Autodesk Inventor part; units mm, degrees
ref_plane "Start plane" through (0, 0, 0) normal (0, 0, 1) x (1, 0, 0)
ref_plane "End plane" through (0, 0, 558.8) normal (0, 0, 1) x (1, 0, 0)
ref_plane "Work Plane4" through (1101.598, 19.05, 0) normal (0.7071, 0, 0.7071) x (0.7071, 0, -0.7071)
ref_plane "Start plane" through (0, 0, 0) normal (0, 0, 1) x (1, 0, 0)
ref_plane "End plane" through (0, 0, 558.8) normal (0, 0, 1) x (1, 0, 0)
sketch "Sketch" plane through (0, 0, 0) normal (0, 0, 1) x (1, 0, 0)
  line L0 (38.1, 0) -> (0, 0)
  line L1 (0, 0) -> (0, 38.1)
  line L2 (0, 38.1) -> (2.4765, 38.1)
  line L3 (4.7625, 35.814) -> (4.7625, 9.5885)
  line L4 (9.5885, 4.7625) -> (35.814, 4.7625)
  line L5 (38.1, 2.4765) -> (38.1, 0)
  line L6 (0, -11.0414) -> (0, 31.5385) construction
  line L7 (-11.0414, 0) -> (31.5385, 0) construction
  arc A0 (4.7625, 9.5885) -> (9.5885, 4.7625) centre (9.5885, 9.5885) ccw
  arc A1 (4.7625, 35.814) -> (2.4765, 38.1) centre (2.4765, 35.814) ccw
  arc A2 (38.1, 2.4765) -> (35.814, 4.7625) centre (35.814, 2.4765) ccw
  line L8 (0, 48.4964) -> (0, -20.9644) construction
  line L9 (-20.9644, 0) -> (48.4964, 0) construction
  point P0 (4.7625, 38.1)
  point P1 (4.7625, 4.7625)
  point P2 (38.1, 4.7625)
  dimension "d0" = 38.1
  dimension "d1" = 38.1
  dimension "d2" = 4.7625
  dimension "d3" = 4.7625
  dimension "d10" = 0
  dimension "d11" = 0
  dimension "d14" = 4.826
  dimension "d15" = 2.286
extrude "Body" add sketch "Sketch" along normal up to surface (558.8 mm away) from surface at 0
sketch "Sketch3" plane through (0, 0, 0) normal (0, 0, 1) x (1, 0, 0)
  line L0 (0, 0) -> (10, 0)
ref_plane "Work Plane3" through (0, 0, 0) normal (0, -1, 0) x (1, 0, 0)
sketch "Sketch4" plane through (0, 0, 0) normal (0, -1, 0) x (1, 0, 0)
  line L0 (-2, 0) -> (12, 0)
  line L1 (-2, 558.8) -> (12, 558.8)
  dimension "d17" = 558.8
ref_plane "Work Plane4" through (1101.598, 19.05, 0) normal (0.7071, 0, 0.7071) x (0.7071, 0, -0.7071)
ref_plane "Work Plane5" through (-130.302, 19.05, 0) normal (-0.7071, 0, 0.7071) x (0.7071, 0, 0.7071)
ref_plane "Work Plane6" through (485.648, 0, 0) normal (-1, 0, 0) x (0, 0, 1)
sketch "Sketch5" plane through (485.648, 0, 0) normal (-1, 0, 0) x (0, 0, 1)
  line L0 (38.1, 0) -> (0, 0)
  line L1 (0, 0) -> (0, 38.1)
  line L2 (0, 38.1) -> (2.4765, 38.1)
  arc A0 (4.7625, 35.814) -> (2.4765, 38.1) centre (2.4765, 35.814) ccw
  line L3 (4.7625, 35.814) -> (4.7625, 9.5885)
  arc A1 (4.7625, 9.5885) -> (9.5885, 4.7625) centre (9.5885, 9.5885) ccw
  line L4 (9.5885, 4.7625) -> (35.814, 4.7625)
  arc A2 (38.1, 2.4765) -> (35.814, 4.7625) centre (35.814, 2.4765) ccw
  line L5 (38.1, 2.4765) -> (38.1, 0)
extrude "Extrusion2" cut sketch "Sketch5" along normal up to surface from surface at -615.95 surface through (-130.302, 19.05, 0) normal (-0.7071, 0, 0.7071)
ref_plane "Work Plane7" through (1101.598, 19.05, 558.8) normal (0.7071, 0, -0.7071) x (0, 1, 0)
ref_plane "Work Plane8" through (-130.302, 19.05, 558.8) normal (-0.7071, 0, -0.7071) x (0, 1, 0)
ref_plane "Work Plane9" through (485.648, 0, 558.8) normal (-1, 0, 0) x (0, 1, 0)
sketch "Sketch6" plane through (485.648, 0, 558.8) normal (-1, 0, 0) x (0, 1, 0)
  line L0 (38.1, 0) -> (0, 0)
  line L1 (0, 0) -> (0, 38.1)
  line L2 (0, 38.1) -> (2.4765, 38.1)
  arc A0 (4.7625, 35.814) -> (2.4765, 38.1) centre (2.4765, 35.814) ccw
  line L3 (4.7625, 35.814) -> (4.7625, 9.5885)
  arc A1 (4.7625, 9.5885) -> (9.5885, 4.7625) centre (9.5885, 9.5885) ccw
  line L4 (9.5885, 4.7625) -> (35.814, 4.7625)
  arc A2 (38.1, 2.4765) -> (35.814, 4.7625) centre (35.814, 2.4765) ccw
  line L5 (38.1, 2.4765) -> (38.1, 0)
extrude "Extrusion3" cut sketch "Sketch6" along normal up to surface from surface at -615.95 surface through (-130.302, 19.05, 558.8) normal (-0.7071, 0, -0.7071)
equation "\"d0\" = G_H"
equation "\"d1\" = G_H"
equation "\"d2\" = G_T"
equation "\"d3\" = G_T"
equation "\"d14\" = G_IR"
equation "\"d15\" = G_ER"
equation "\"d4\" = G_L"
equation "\"G_H\" = 38.1"
equation "\"G_T\" = 4.7625"
equation "\"G_ER\" = 2.286"
equation "\"G_IR\" = 4.826"
equation "\"G_L\" = d17"
equation "\"ex\" = 0"
equation "\"G_OFFSET_START\" = 0"
equation "\"G_OFFSET_END\" = 0"
equation "\"d13\" = G_OFFSET_END + B_L"
equation "\"B_L\" = 558.8"
properties part number "AISC - L 1.5 x 1.5 x 3/16 - 22" material "Aluminum 6061"
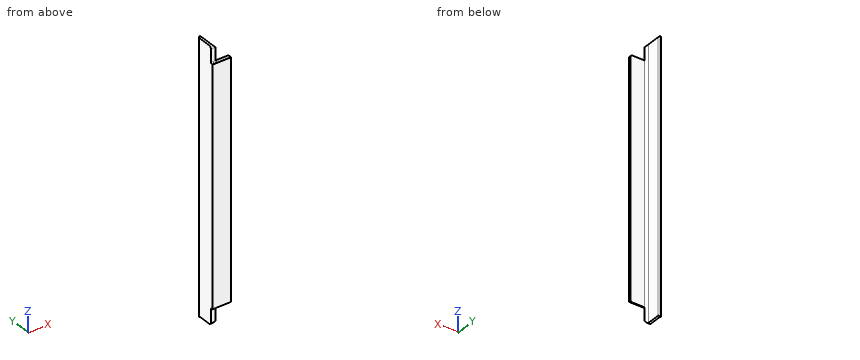
Source: CAD feature listing. Evaluate the final solid. Frame: model axes, mm. Round coordinates to 2 decimals unless told otherwise and drop trailing zeros. Order: outer loops, then holes, each group sorted by start corner. A loop starts at its lowest first (then second) coordinate and runs counter-clockwise, first axis right, second up. Notation, with made-up numbers: (54.25, 25.5) -> (91.25, 25.5) arc R35 cw to (91.25, 59.5) -> close; hole circle Ø2 at (-2.75, -2.5). An arc over 180 degrees is marked (long way). Use CSV: the item, a comma, the result in double quotes.
(1) Section B-B on x = 29. Return the cut outline in (y, z), and give its area (3 significant figures).
Report:
outline,"(0, 38.1) -> (2.48, 38.1) arc R2.29 cw to (4.76, 35.81) -> (4.76, 522.99) arc R2.29 cw to (2.48, 520.7) -> (0, 520.7) -> close"
area,"2,300 mm^2"
(2) Section C-C on y = 28. Return the cut outline in (x, z).
Report:
outline,"(0, 4.76) -> (4.76, 4.76) -> (4.76, 554.04) -> (0, 554.04) -> close"
(3) Section A-A on z = 362.5. Return the cut outline in (x, y).
Report:
outline,"(0, 0) -> (38.1, 0) -> (38.1, 2.48) arc R2.29 ccw to (35.81, 4.76) -> (9.59, 4.76) arc R4.83 cw to (4.76, 9.59) -> (4.76, 35.81) arc R2.29 ccw to (2.48, 38.1) -> (0, 38.1) -> close"
(4) First-contact query: pin 1 Ø0.7 at (x, y) = (24.5, 0.5) entering from -Z; pin 2 Ø2 at (y, z) = (17, 215.5) entering from +X; pin 3 Ø5 at (x, z) = (6.5, 531) entering from -Y. Flat tips, straight axial feed; report the tip coordinate or a pass-through.
Report:
pin 1,"z = 38.1"
pin 2,"x = 4.76"
pin 3,"y = 4.76"
(5) Ray query, L1, parallel to X at y = 30.5, z = 27; L2, parallel to X at y = 3.5, z = 517. Return the intervals inside material, ascending.
Report:
L1,"0 to 4.76"
L2,"0 to 37.86"
